from build123d import *

# Parameters (mm, degrees)
SKETCH2_R           = 3.175
SKETCH2_R_2         = 2.0399375
BOSS_EXTRUDE1_DEPTH = 2.38125
SKETCH2_6_R         = 3.175
SKETCH2_6_R_2       = 2.0399375
BOSS_EXTRUDE2_DEPTH = 3.175
CUT_EXTRUDE1_START  = -0.79375
SKETCH3_R           = 3.571875
SKETCH3_R_2         = 2.0399375
CUT_EXTRUDE1_DEPTH  = 0.79375
FILLET1_START       = 1.5875
FILLET1_DEPTH       = 0.79375


with BuildPart() as part:
    # Sketch2 → Boss-Extrude1 (new body)
    with BuildSketch(Plane.XY):
        with BuildLine():
            ThreePointArc((-4.001636369, -3.854714053), (-3.061446657, -5.68510333), (-3.28705844, -7.730434825))
            ThreePointArc((-3.28705844, -7.730434825), (3.2e-08, -12.7), (3.287058415, -7.730434766))
            ThreePointArc((3.287058415, -7.730434766), (3.061446657, -5.685103331), (4.001636324, -3.8547141))
            ThreePointArc((4.001636324, -3.8547141), (3.3e-08, 5.55625), (-4.001636369, -3.854714053))
        make_face()
        Circle(SKETCH2_R, mode=Mode.SUBTRACT)
        with Locations((0, -9.128125)):
            Circle(SKETCH2_R_2, mode=Mode.SUBTRACT)
    extrude(amount=BOSS_EXTRUDE1_DEPTH)

    # Sketch2<6> → Boss-Extrude2 (add)
    with BuildSketch(Plane.XY):
        Circle(SKETCH2_6_R)
        Circle(SKETCH2_6_R_2, mode=Mode.SUBTRACT)
    extrude(amount=BOSS_EXTRUDE2_DEPTH)

    # Sketch3 → Cut-Extrude1 (cut)
    with BuildSketch(Plane.XY.offset(2.38125).offset(CUT_EXTRUDE1_START)):
        with Locations((0, -9.128125)):
            Circle(SKETCH3_R)
        with Locations((0, -9.128125)):
            Circle(SKETCH3_R_2, mode=Mode.SUBTRACT)
    extrude(amount=CUT_EXTRUDE1_DEPTH, mode=Mode.SUBTRACT)

    # Fillet1: read off the stored shape, not the designer's step
    # Fillet1 outline → Fillet1 (cut)
    with BuildSketch(Plane.XY.offset(FILLET1_START)):
        with BuildLine():
            ThreePointArc((-3.287058422, -7.730434783), (-2.475434769, -6.553146608), (-1.267079181, -5.788543984))
            ThreePointArc((-1.267079181, -5.788543984), (-2.451421136, -5.765200609), (-3.289884364, -4.928426927))
            ThreePointArc((-3.289884364, -4.928426927), (-3.002243662, -6.329142182), (-3.287058422, -7.730434783))
        make_face()
        with BuildLine():
            ThreePointArc((3.289884364, -4.928426927), (2.451421136, -5.765200609), (1.267079181, -5.788543984))
            ThreePointArc((1.267079181, -5.788543984), (2.475434769, -6.553146608), (3.287058422, -7.730434783))
            ThreePointArc((3.287058422, -7.730434783), (3.002243662, -6.329142182), (3.289884364, -4.928426927))
        make_face()
    extrude(amount=FILLET1_DEPTH, mode=Mode.SUBTRACT)


solid = part.part
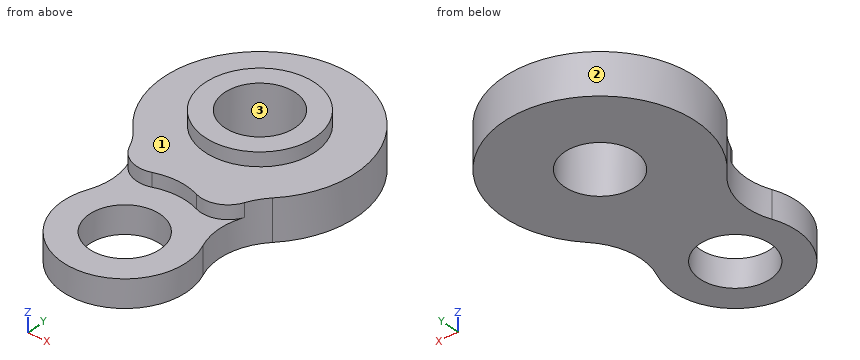
Design review of the part built by this model. Coordinates are the model's own, in mm. Face numbers are marked on the shaded views. Round coordinates to 2 decimals unless told otherwise and drop trailing zeros. Write each loop counter-clockwise with the first axis right and the second up, starting at its lowest first coordinate (ties: lowest second). Pieces come first, ordered by that corner, then holes. Notation, with made-up numbers: (-14.75, 59.5) - (34.25, 59.5) arc R23 ccw to (34.25, 89.5) - close; hole circle Ø9 at (1.25, 14). An arc over 180 degrees is marked (long way). Use a Markdown table: item, result. Add a question column.
1. Clearance check with flat-ended pins moving along their axes: pin 1 (2 mm diameter, centred on x = 1, y = -7, fed in from +Z); pin 2 (2.5 mm diameter, centred on x = 0, y = 0, fed in from -Z). State where each tip first meets the part, or that it passes through.
2. We need section C-C (y = 0). State the section outline as (x, z) points (3 decimals).
3. We need section A-A (x = 0). State the section outline as (y, z) points (1 decimal).
4. We need section D-D (z = 0.5). State the section outline as (x, y) points, then the cut area to 3 significant figures.
5. Wall thickness on probe 1 along Y at (x, z) = (1.75, 0.4); probe 2 along Y at (x, z) = (0, 2.45) (3 decimals); probe 3 along Z at (x, y) = (-1.5, -3.25): over which ranges is each line inside the solid? List them lowest first.
6. Mouldability with a two-part tool opening along X and no side actions: class the marked faces 1, 2 and 3 as +X half, -X half, draft (parallel to the pull), parting line (faces both ways), or undercut.
7. We need section B-B (z = 2.2). State the section outline as (x, y) points (1 decimal), then the cut area to 3 significant figures.
Output:
| question | item | result |
|---|---|---|
| 1 | pin 1 | stops at z = 1.59 |
| 1 | pin 2 | passes through |
| 2 | outline | (-5.556, 0) - (-2.04, 0) - (-2.04, 3.175) - (-3.175, 3.175) - (-3.175, 2.381) - (-5.556, 2.381) - close; (2.04, 0) - (5.556, 0) - (5.556, 2.381) - (3.175, 2.381) - (3.175, 3.175) - (2.04, 3.175) - close |
| 3 | outline | (-12.7, 0) - (-11.2, 0) - (-11.2, 1.6) - (-12.7, 1.6) - close; (-7.1, 0) - (-2, 0) - (-2, 3.2) - (-3.2, 3.2) - (-3.2, 2.4) - (-5.6, 2.4) - (-5.6, 1.6) - (-7.1, 1.6) - close; (2, 0) - (5.6, 0) - (5.6, 2.4) - (3.2, 2.4) - (3.2, 3.2) - (2, 3.2) - close |
| 4 | outline | (-4, -3.85) arc R3.57 cw to (-3.29, -7.73) arc R3.57 ccw (long way) to (3.29, -7.73) arc R3.57 cw to (4, -3.85) arc R5.56 ccw (long way) to start; hole circle Ø4.08 at (0, -9.13); hole circle Ø4.08 at (0, 0) |
| 4 | area | 116 mm2 |
| 5 | probe 1 | y = -12.24 to -10.18, -8.08 to -1.05, 1.05 to 5.27 |
| 5 | probe 2 | y = -3.175 to -2.04, 2.04 to 3.175 |
| 5 | probe 3 | z = 0 to 2.38 |
| 6 | face 1 | draft |
| 6 | face 2 | parting line |
| 6 | face 3 | undercut |
| 7 | outline | (-4, -3.9) arc R3.6 cw to (-3.3, -4.9) arc R1.6 ccw to (-1.3, -5.8) arc R3.6 cw to (1.3, -5.8) arc R1.6 ccw to (3.3, -4.9) arc R3.6 cw to (4, -3.9) arc R5.6 ccw (long way) to start; hole circle Ø4.1 at (0, 0) |
| 7 | area | 87.1 mm2 |
